```python
from build123d import *

# Parameters (mm, degrees)
BOSS_EXTRUDE1_DEPTH      = 15
BOSS_EXTRUDE1_DEPTH_BACK = 15
SKETCH1_R                = 9.12611675
SKETCH1_R_2              = 6.232505418


with BuildPart() as part:
    # Sketch1 → Boss-Extrude1 (new, two sides: drawn at the far end of the back side and taken through both)
    with BuildSketch(Plane(origin=(0, 0, 0), x_dir=(1, 0, 0), z_dir=(0, 1, 0)).offset(-BOSS_EXTRUDE1_DEPTH_BACK)):
        with BuildLine():
            Line((-194.484920724, -50.304604359), (-148.298710109, -50.304604359))
            ThreePointArc((-148.298710109, -50.304604359), (-124.484920724, -32.914035031), (-100.67113134, -50.304604359))
            Line((-100.67113134, -50.304604359), (205.515079276, -45.523465704))
            Line((205.515079276, -45.523465704), (205.515079276, -65.523465704))
            Line((205.515079276, -65.523465704), (-100.67113134, -65.523465704))
            ThreePointArc((-100.67113134, -65.523465704), (-124.484920724, -82.914035031), (-148.298710109, -65.523465704))
            Line((-148.298710109, -65.523465704), (-194.484920724, -65.523465704))
            Line((-194.484920724, -65.523465704), (-194.484920724, -50.304604359))
        make_face()
        with Locations(Location((-124.484920724, -57.914035031, 0), (0, 0, 270))):
            Circle(SKETCH1_R, mode=Mode.SUBTRACT)
        with Locations(Location((-181.826571095, -57.914035031, 0), (0, 0, 270))):
            Circle(SKETCH1_R_2, mode=Mode.SUBTRACT)
    extrude(amount=BOSS_EXTRUDE1_DEPTH + BOSS_EXTRUDE1_DEPTH_BACK)


solid = part.part
```
Build history of the part. All positions in model axes, mm. A direction names the side the tool comes from. Give positions to 0.01 mm unless a question says otherwise; leave off trailing zeros. Order: outer loops, then holes, each group sorted by start corner. A loop starts at its lowest first (then second) coordinate and runs counter-clockwise, first axis right, second up. Notation, with made-up numbers: M -18,67.5 L -11,67.5 A9 cw -11,78.5 Z; hole C 8,-7 d7. An arc over 180 degrees is marked long. Write item = value, one per line. Start each with the question number.
(1) Slice it at B-B on y = 10. Write the cut outline in (x, z), plus the area to 3 significant figures.
(2) Which spindle directions (+Z, -Z, +X, -X, +Y, -Y) get a long thin tool onto all of the face, cutting with end or side? Do faces 1 (the flat face through (55, 0, 65.523)), 2 (the flat face through (8, -15, 58)), 3 (the flat face through (-171, 0, 65.523)). Say none if no direction does.
(3) Slice it at C-C on x = -163. Write the cut outline in (y, z).
(4) Pin check, flat tips, straight feed: pin 1 Ø2 at (y, z) = (0.5, 47.5) entering from -X; pin 2 Ø2 at (x, y) = (-114, 7.5) entering from +Z; pin 3 Ø14.5 at (x, z) = (-124.48, 57.91) entering from -Y; pin 4 Ø15 at (x, y) = (85, -2.5) entering from +Z. Stop position of each tip, or through.
(5) Slice it at A-A on z = 60.5. Write the cut outline in (x, y).
(6) Two-plate mould, pull along X, no slides. Class faces 4 (the cylindrical face through (-124.04, -0.21, 82.91)), 5 (the flat face through (-172, 0, 50.305)), 6 (the cylindrical face through (-187.91, -0.21, 56.56)), 7 (the cylindrical face through (-133.394, -0.21, 55.936)): released by +X, released by -X, zero draft, split by the parting line, or undercut.
(7) Probe L1, parallel to Z at x = -171, y = -8.25; L2, parallel to X at y = 0.5, z = 61; L3, parallel to Z at x = -3, y = -0.5. List the from-to ranges inside material, lowest first. Write a range as [from, to].
(8) Slice it at D-D on x = 165.5. Write the cut outline in (y, z), plus the area to 3 significant figures.
Responses:
q1.outline = M -194.48,50.3 L -148.3,50.3 A25 ccw -100.67,50.3 L 205.52,45.52 L 205.52,65.52 L -100.67,65.52 A25 ccw -148.3,65.52 L -194.48,65.52 Z; hole C -181.83,57.91 d12.47; hole C -124.48,57.91 d18.25
q1.area = 7,650 mm2
q2.face_1 = +Z, +X, +Y, -Y
q2.face_2 = +Z, -Z, +X, -X, -Y
q2.face_3 = +Z, -X, +Y, -Y
q3.outline = M -15,50.3 L 15,50.3 L 15,65.52 L -15,65.52 Z
q4.pin_1 = -147.64
q4.pin_2 = 81.04
q4.pin_3 = through
q4.pin_4 = 65.52
q5.outline = M -194.48,-15 L -187.5,-15 L -187.5,15 L -194.48,15 Z; M -176.16,-15 L -133.24,-15 L -133.24,15 L -176.16,15 Z; M -115.73,-15 L 205.52,-15 L 205.52,15 L -115.73,15 Z
q6.face_4 = split by the parting line
q6.face_5 = zero draft
q6.face_6 = undercut
q6.face_7 = undercut
q7.L1 = [50.3, 65.52]
q7.L2 = [-194.48, -187.24], [-176.41, -133.07], [-115.9, 205.52]
q7.L3 = [48.78, 65.52]
q8.outline = M -15,46.15 L 15,46.15 L 15,65.52 L -15,65.52 Z
q8.area = 581 mm2
